For this review, use the dimensioned drawing (mm, ordinates from the lowest corner) and the shaded views. A direction names the side the tool comes from. Coordinates: 2 decimals unless noted, no trailing zeros. Write each loop counter-clockwise with the first axis right and the second up, starting at its lowest first coordinate (ties: lowest second). Pieces come first, ordered by that corner, then holes. Notation, with made-up numbers: M 13,-18 L 58,-18 A20 ccw 58,-14 Z; hole C 67,60 d6. An arc over 180 degrees is marked long. One line per question, with ' | ' between items.
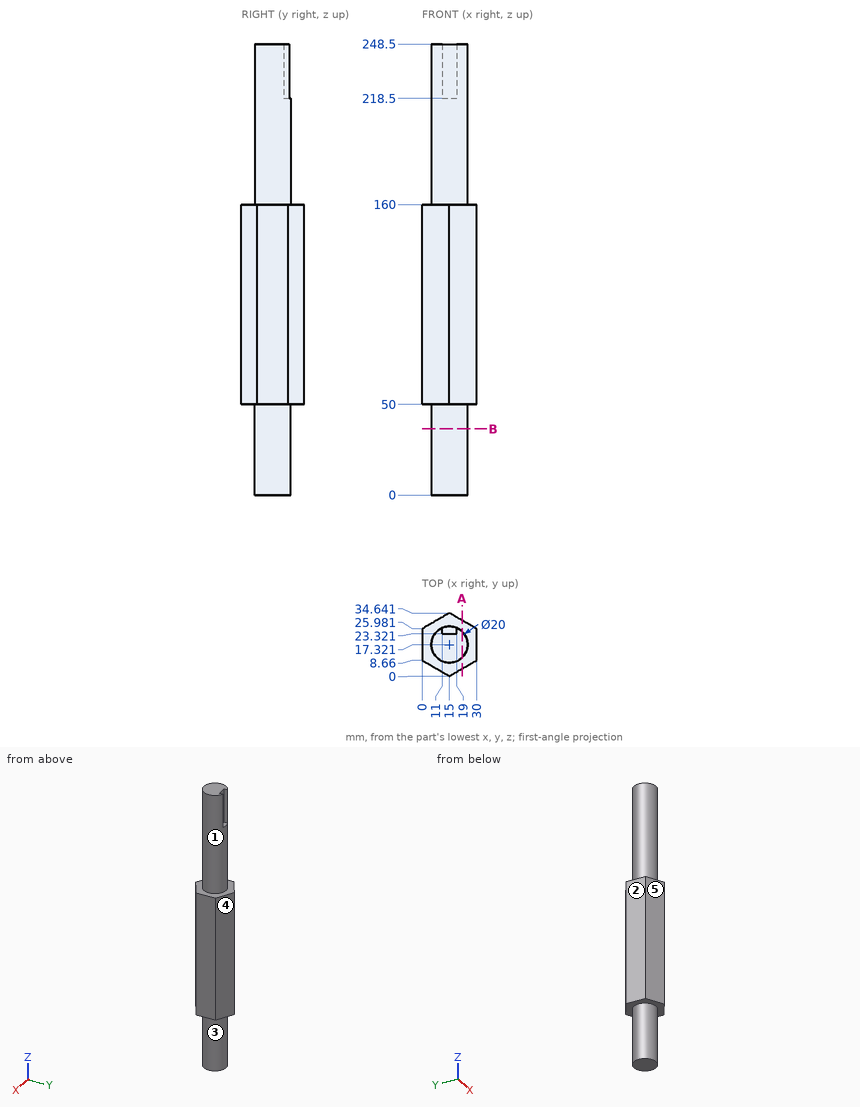
1. Tool access review of the marked faces 1 and 2: name each direction out of +Z, -Z, +X, -X, +Y, -Y from which nothing blocks a thin tool from reaching the whole face with its end or side.
Answer sheet:
face 1: +Z | face 2: +Z, -Z, -X, +Y, -Y
2. Take a section at A-A (x = 22). Write out the cut boundary in (y, z).
Answer sheet:
outline: M 4.04,50 L 10.18,50 L 10.18,0 L 24.46,0 L 24.46,50 L 30.6,50 L 30.6,160 L 24.46,160 L 24.46,248.5 L 10.18,248.5 L 10.18,160 L 4.04,160 Z
3. Take a section at B-B (z = 36.5). Write out the cut boundary in (x, y), then the cut area to 3 significant figures.
Answer sheet:
outline: C 15,17.32 d20 | area: 314 mm^2
4. To check wall thickness, follow line 1 along Z through (x, y) = (4.75, 14); line 2 along X through (y, z) = (17, 170.5) (1 decimal); line 3 along Y through (x, z) = (2.25, 147). State the ranges of each line that lie inside material, in increasing order. Write a range as [from, to].
Answer sheet:
line 1: [50, 160] | line 2: [5, 25] | line 3: [7.36, 27.28]
5. Draft analysis for pull direction X (two halves, no side actions). For the marked faces 3, 4 and 5, state which applies: pulls with the +X half, pulls with the -X half, needs draft (parallel to the pull), parting line crosses it, or undercut.
Answer sheet:
face 3: parting line crosses it | face 4: pulls with the +X half | face 5: pulls with the -X half
6. Insertion check: pin 1 Ø3 at (x, y) = (15.5, 25) entering from +Z; pin 2 Ø2 at (x, y) = (13, 17) entering from -Z; pin 3 Ø1.5 at (x, z) = (14, 216) entering from -Y; pin 4 Ø2 at (y, z) = (23.5, 42) entering from +X (1 decimal). Each pin has a flat end and moves straight along its axis. Give the tip position at first contact, or say it passes through.
Answer sheet:
pin 1: z = 218.5 | pin 2: z = 0 | pin 3: y = 7.32 | pin 4: x = 23.6
